```python
from build123d import *

# Parameters (mm, degrees)
F0_W     = 63.5
F0_H     = 63.5
F1_DEPTH = 25.4
F2_R     = 21.59
F3_DEPTH = 53.34
F4_R     = 4.572
F5_DEPTH = 6.35
F7_DEPTH = 5.08
F8_DEPTH = 5.08


with BuildPart() as f1:
    # F0 (on Top) → F1 (new body)
    with BuildSketch(Plane.XY):
        Rectangle(F0_W, F0_H)
    extrude(amount=F1_DEPTH)

    # F2 (on face) → F3 (cut)
    with BuildSketch(Plane.YZ.offset(31.75)):
        with Locations((0, 25.4)):
            Circle(F2_R)
    extrude(amount=-F3_DEPTH, mode=Mode.SUBTRACT)

    # F4 (on face) → F5 (join)
    with BuildSketch(Plane(origin=(0, 0, 0), x_dir=(1, 0, 0), z_dir=(0, 0, -1))):
        with Locations((26.67, 0)):
            Circle(F4_R)
    extrude(amount=F5_DEPTH)

    # F6 (on face) → F7 (cut)
    with BuildSketch(Plane.YZ.offset(-21.59)):
        with BuildLine():
            Line((-2.54, 8.89), (-2.54, 3.9599323695))
            ThreePointArc((-2.54, 3.9599323695), (0, 3.81), (2.54, 3.9599323695))
            Line((2.54, 3.9599323695), (2.54, 8.89))
            Line((2.54, 8.89), (13.9121529606, 8.89))
            ThreePointArc((13.9121529606, 8.89), (0, 46.99), (-13.9121529606, 8.89))
            Line((-13.9121529606, 8.89), (-2.54, 8.89))
        make_face()
    extrude(amount=-F7_DEPTH, mode=Mode.SUBTRACT)

    # F6 (on face) → F8 (cut)
    with BuildSketch(Plane.YZ.offset(-21.59)):
        with BuildLine():
            Line((-2.54, 8.89), (-2.54, 3.9599323695))
            ThreePointArc((-2.54, 3.9599323695), (0, 3.81), (2.54, 3.9599323695))
            Line((2.54, 3.9599323695), (2.54, 8.89))
            Line((2.54, 8.89), (13.9121529606, 8.89))
            ThreePointArc((13.9121529606, 8.89), (0, 46.99), (-13.9121529606, 8.89))
            Line((-13.9121529606, 8.89), (-2.54, 8.89))
        make_face()
    extrude(amount=-F8_DEPTH, mode=Mode.SUBTRACT)


solid = f1.part
```
Design review of the part built by this model. Coordinates are the model's own, in mm. A direction names the side the tool comes from. Give positions to 0.01 mm unless a question says otherwise; leave off trailing zeros. Order: outer loops, then holes, each group sorted by start corner. A loop starts at its lowest first (then second) coordinate and runs counter-clockwise, first axis right, second up. Notation, with made-up numbers: (71.5, -19.5) - (99.5, -19.5) arc R25 ccw to (99.5, 3.5) - close; hole circle Ø10 at (-39, 88). An arc over 180 degrees is marked (long way). Use a Markdown table: item, result. Add a question column.
(1) Add section B-B on y = 0. Give the boundary of the cut face in (x, z).
(2) Add section D-D on x = -3. Give the boundary of the cut face in (y, z), then the cut area to 3 significant figures.
(3) Wall thickness on probe 1 along X at (y, z) = (2, 17); probe 2 along Y at (x, z) = (25, 13.5); probe 3 along Z at (x, y) = (-19, 25.5): over which ranges is each line inside the solid? List them lowest first. Write a range as [from, to].
(4) Add section C-C on z = -4. Give the boundary of the cut face in (x, y), then the cut area to 3 significant figures.
(5) Add section A-A on x = 26.67. Give the boundary of the cut face in (y, z).
(6) Machinability: for faces 5 (the face through (-21.59, -7, 7)), 6 (the face through (-8, 22, 25.4)), which of the approach directions +Z, -Z, +X, -X, +Y, -Y give a long, thin tool a straight path to every point of the face, cutting with its end or side? Answer none if there is none.
(7) Mouldability with a two-part tool opening along Y and no side actions: class faces 1 (the face through (30.893, 1.751, -3.131)), 2 (the face through (-24, 8, 8.89)), 3 (the face through (0, -31.75, 13)), 4 (the face through (0, 0, 0)) as +Y half, -Y half, draft (parallel to the pull), parting line (faces both ways), or undercut.
(8) Clearance check with flat-ended pins moving along their axes: P1, Ø1.5, axis at x = -24, y = -8, coming from the +Z side; P2, Ø5, axis at x = -2, z = -3, coming from the -Y side; P3, Ø1.5, axis at y = 4.5, z = 10.5, coming from the +X side; P4, Ø3, axis at x = 3.5, y = 17, coming from the +Z side. State where each tip first meets the part, or that it passes through.
Report:
| question | item | result |
|---|---|---|
| 1 | outline | (-31.75, 0) - (22.1, 0) - (22.1, -6.35) - (31.24, -6.35) - (31.24, 0) - (31.75, 0) - (31.75, 3.81) - (-26.67, 3.81) - (-26.67, 25.4) - (-31.75, 25.4) - close |
| 2 | outline | (-31.75, 0) - (31.75, 0) - (31.75, 25.4) - (21.59, 25.4) arc R21.59 cw to (-21.59, 25.4) - (-31.75, 25.4) - close |
| 2 | area | 881 mm² |
| 3 | probe 1 | x = [-31.75, -26.67] |
| 3 | probe 2 | y = [-31.75, -18.01], [18.01, 31.75] |
| 3 | probe 3 | z = [0, 25.4] |
| 4 | outline | circle Ø9.14 at (26.67, 0) |
| 4 | area | 65.7 mm² |
| 5 | outline | (-31.75, 0) - (-4.57, 0) - (-4.57, -6.35) - (4.57, -6.35) - (4.57, 0) - (31.75, 0) - (31.75, 25.4) - (21.59, 25.4) arc R21.59 cw to (-21.59, 25.4) - (-31.75, 25.4) - close |
| 6 | face 5 | +Z, +X |
| 6 | face 6 | +Z, +X, -X, +Y, -Y |
| 7 | face 1 | parting line |
| 7 | face 2 | undercut |
| 7 | face 3 | -Y half |
| 7 | face 4 | draft |
| 8 | P1 | stops at z = 8.89 |
| 8 | P2 | passes through |
| 8 | P3 | stops at x = -26.67 |
| 8 | P4 | stops at z = 14.27 |
